Part model, mm, in its own coordinate system. A direction names the side the tool comes from. Round coordinates to 2 decimals unless told otherwise and drop trailing zeros. Write each loop counter-clockwise with the first axis right and the second up, starting at its lowest first coordinate (ties: lowest second). Pieces come first, ordered by that corner, then holes.
Autodesk Inventor part; units mm, degrees
ref_plane "YZ Plane" through (0, 0, 0) normal (1, 0, 0) x (0, 1, 0)
ref_plane "XZ Plane" through (0, 0, 0) normal (0, 1, 0) x (-1, 0, 0)
ref_plane "XY Plane" through (0, 0, 0) normal (0, 0, 1) x (1, 0, 0)
sketch "スケッチ1" plane through (0, 0, 0) normal (0, 1, 0) x (-1, 0, 0)
  circle A0 centre (0, 0) radius 1.15
  circle A1 centre (0, 0) radius 2
  circle A2 centre (0, 0) radius 5
  line L0 (0, 0) -> (7, 0)
  line L1 (7, 0) -> (7, 4.5)
  line L2 (7, 4.5) -> (0, 4.5)
  line L3 (0, 4.5) -> (0, 0)
  line L4 (0, 0) -> (7, 0)
  line L5 (7, 0) -> (7, -5)
  line L6 (7, -5) -> (0, -5)
  line L7 (0, -5) -> (0, 0)
  line L8 (0, 4.5) -> (-2, 4.5)
  line L9 (-2, 4.5) -> (-2, 0)
  line L10 (-2, 0) -> (0, 0)
  line L11 (0, 0) -> (0, 4.5)
  circle A3 centre (0, 0) radius 3
  line L12 (-2, 0) -> (-2, -5)
  line L13 (-2, -5) -> (0, -5)
  line L14 (2, 0) -> (2, -5)
  circle A4 centre (0, 0) radius 4.9244
  line L15 (-2, 0) -> (-4.9244, 0)
  line L16 (0, -4.9244) -> (0, -5.9244)
  line L17 (0, -5.9244) -> (7, -5.9244)
  line L18 (7, -5.9244) -> (7, -5)
  line L19 (7, -5) -> (0, -5.9244)
  line L20 (0, -5.9244) -> (4.9138, -5)
  point P0 (0, 2)
  point P1 (-2, 2.2361)
  point P2 (-2, -2.2361)
  point P3 (-2, -4.5826)
  point P4 (-2, -4.5)
  point P5 (0, -4.9244)
  dimension "d2" = 10
  dimension "d0" = 2.3
  dimension "d1" = 4
  dimension "d3" = 7
  dimension "d4" = 4.5
  dimension "d5" = 6
  dimension "d22" = 1
  dimension "d34" = 5
extrude "押し出し1" add sketch "スケッチ1" along normal blind 4.5 contours A1 L3 A3 L0 | L0 A3 L14 | A3 L3 L2 A4 L0 | L0 A4 L14 A3 | A4 L2 A2 L0 | L0 A2 L14 A4 | L0 L5 L6 L14 A2 | A2 L2 L1 L0
extrude "押し出し2" add sketch "スケッチ1" along normal blind 3 contours A1 L9 A3 L3 | L15 A3 L9 | L12 A3 L15 | A3 L9 L8 L3 | A3 L15 A4 L9 | L12 A4 L15 A3
extrude "押し出し3" add sketch "スケッチ1" against normal blind 1 contours L0 A1 L7 A0 | A0 L3 A1 L0 | A0 L10 A1 L3 | L7 A1 L10 A0 | L14 A3 L7 A1 | A1 L3 A3 L0 | L0 A3 L14 | A1 L9 A3 L3 | L7 A3 L12 A1 | A3 L3 L2 A4 L0 | L0 A4 L14 A3 | L14 A4 L7 A3 | L15 A3 L9 | L12 A3 L15 | A3 L9 L8 L3 | L7 A4 L12 A3 | A4 L2 A2 L0 | L0 A2 L14 A4 | L14 A2 L7 A4 | A3 L15 A4 L9 | L12 A4 L15 A3 | L0 L5 L6 L14 A2 | A2 L2 L1 L0 | L14 L6 A2 | L6 L20 L16
sketch "スケッチ2" plane through (0, 4.5, 0) normal (0, 1, 0) x (1, 0, 0)
  circle A0 centre (0, 0) radius 1.15
  circle A1 centre (0, 0) radius 2
  circle A2 centre (0, 0) radius 4.9244
  line L0 (0, 0) -> (2, 0)
  line L1 (2, 0) -> (2, -4.5)
  line L2 (2, -4.5) -> (0, -4.5)
  line L3 (0, -4.5) -> (0, 0)
  line L4 (-2, 5) -> (-7, 5)
  line L5 (0, -4.5) -> (-7, -4.5)
  line L6 (-7, -4.5) -> (-7, 5)
  line L7 (-7, 5) -> (0, 5)
  line L8 (0, 5) -> (0, -4.5)
  line L9 (0, 0) -> (2, 0)
  line L10 (2, 0) -> (2, 5)
  line L11 (2, 5) -> (0, 5)
  line L12 (0, 5) -> (0, 0)
  line L13 (0, 5) -> (-7, 5)
  line L14 (0, 5.9244) -> (0, 5)
  line L15 (-7, 5) -> (0, 5.9244)
  line L16 (0, 5.9244) -> (-4.9138, 5)
  line L17 (-2, 5) -> (-7, 5)
  point P0 (0, 4.9244)
  dimension "d12" = 4
  dimension "d35" = 5
extrude "押し出し4" add sketch "スケッチ2" along normal blind 1 contours L0 A1 L3 A0 | A0 L8 A1 L0 | A0 L3 A1 L8 | L1 L2 L3 A1 | L10 A2 L1 | A1 L8 A2 L10 | A1 L3 L5 A2 L8 | A2 L5 L6 L4 L7 L8 | L7 L4 L16 L14
sketch "スケッチ4" plane through (0, 3, 4.5) normal (0, 0, 1) x (1, 0, 0)
  line L0 (-7, 2.5) -> (2, 2.5)
  line L1 (-7, 2.5) -> (-4.5, 2.5)
  line L2 (-4.5, 2.5) -> (-4.5, -0.75)
  line L3 (-4.5, -0.75) -> (-7, -0.75)
  line L4 (-7, -0.75) -> (-7, 2.5)
  circle A0 centre (-4.5, -0.75) radius 1.4
  line L5 (0, -3) -> (0, -2.5)
  line L6 (0, -2.5) -> (-1.5, -2.5)
  circle A1 centre (-1.5, -2.5) radius 0.5
  dimension "d23" = 2.5
  dimension "d24" = 3.25
  dimension "d25" = 2.8
  dimension "d26" = 0.5
  dimension "d27" = 1.5
  dimension "d28" = 1
extrude "押し出し6" cut sketch "スケッチ4" against normal blind 6 contours A0 L3 L2 | L2 L3 A0 | A1
chamfer "面取り2" distance 2 angle 45 3 edges at (-7, 5.5, -0.25) (-7, -1, -0.25) (-7, 2.25, -5)
properties part number "rod5.5"
Q1. Saw through at D-D, the plane x = -2.25. Write the cut outline in (y, z), and give its area (3 significant figures).
Q2. Saw through at C-C, the plane y = -0.5. Write the cut outline in (x, z).
Q3. Tool access for faces 4 (the flat face through (-2, 2, -2)), 5 (the flat face through (1, 4.5, -1)), 6 (the flat face through (0, 5, -5.4)), 7 (the flat face through (2, 3, 1)): list every direction of +Z, -Z, +X, -X, +Y, -Y with a clear straight run to the whole face (end or side of a thin tool).
Q4. Wall check: line 1 (Y direction, x = -1.5, z = -3); line 2 (Y direction, x = 2.5, z = 3); line 3 (X direction, y = -0.6, z = 0). Give the ranges that are in metal, low to high.
Q5. Saw through at B-B, the plane x = 2.5. Write the cut outline in (y, z), and give its area (3 significant figures).
Q6. Two-plate mould, pull along Y, no slides. Class faces 1 (the cylindrical face through (4.8, 5, -1.1)), 2 (the flat face through (-6, 4.5, -0.2)), 3 (the cylindrical face through (-3.85, 1.01, 1.54)): released by +Y, released by -Y, zero draft, split by the parting line, or undercut.
Q7. Drop flat-ended pins along their axis: P1, Ø1.6, axis at y = 3.5, z = 3.5, coming from the +X side; P2, Ø2, axis at x = -4.5, y = 2.25, coming from the +Z side; P3, Ø2, axis at y = 3, z = -2, coming from the +X side. Give the stop position or say it passes through.
Q8. Saw through at A-A, the plane z = 0.5. Write the cut outline in (x, y), and give its area (3 significant figures).
Computed:
1. outline: (-1, -5.5) - (0, -5.5) - (0, -5) - (4.5, -5) - (4.5, -5.5) - (5.5, -5.5) - (5.5, 4.5) - (-1, 4.5) - close
1. area: 62.8 mm2
2. outline: (-5.5, -4.5) - (-5, -5) - (-4.91, -5) - (0, -5.92) - (0, -4.92) arc R4.92 ccw to (2, 4.5) - (-5.5, 4.5) - close; hole circle Ø2.3 at (0, 0)
3. face 4: -Z
3. face 5: -Z, +X
3. face 6: -Z, +X, +Y, -Y
3. face 7: +Z, -Z, +X
4. line 1: y = -1 to 0, 4.5 to 5.5
4. line 2: y = -1 to 3, 4.5 to 5.5
4. line 3: x = -5.4 to -1.15, 1.15 to 4.92
5. outline: (-1, -4.24) - (3, -4.24) - (3, 4.24) - (-1, 4.24) - close; (4.5, -4.24) - (5.5, -4.24) - (5.5, 4.24) - (4.5, 4.24) - close
5. area: 42.4 mm2
6. face 1: zero draft
6. face 2: released by +Y
6. face 3: undercut
7. P1: stops at x = 4
7. P2: stops at z = -1.5
7. P3: stops at x = 4.82
8. outline: (-7, 1) - (-5, -1) - (-1.04, -1) - (-1.04, 0) - (-1.94, 0) - (-1.94, 0.26) arc R0.5 cw to (-1.94, 0.74) - (-1.94, 4.5) - (-1.04, 4.5) - (-1.04, 5.5) - (-5, 5.5) - (-7, 3.5) - close; (1.04, -1) - (4.9, -1) - (4.9, 3) - (1.94, 3) - (1.94, 0) - (1.04, 0) - close; (1.04, 4.5) - (4.9, 4.5) - (4.9, 5.5) - (1.04, 5.5) - close; hole circle Ø2.8 at (-4.5, 2.25)
8. area: 41.2 mm2
